Here's how the part is built. I have some questions about the finished solid (model axes, mm). A direction names the side the tool comes from. Give positions to 0.01 mm unless a question says otherwise; leave off trailing zeros. Loops run counter-clockwise (first coordinate to the right, second up) from the corner with the lowest first, then second, coordinate; pieces in that order, holes last. Notation, with made-up numbers: M -12,18 L 33,18 A21 ccw 33,30 Z; hole C -10,-20.5 d7. An arc over 180 degrees is marked long. Write item = value, one per line. Start each with the question number.
Autodesk Inventor part; units mm, degrees
ref_plane "YZ Plane" through (0, 0, 0) normal (1, 0, 0) x (0, 1, 0)
ref_plane "XZ Plane" through (0, 0, 0) normal (0, 1, 0) x (-1, 0, 0)
ref_plane "XY Plane" through (0, 0, 0) normal (0, 0, 1) x (1, 0, 0)
sketch "Sketch1" plane through (0, 0, 0) normal (0, 0, 1) x (1, 0, 0)
  line L0 (-15.5, -9) -> (15.5, -9)
  line L1 (15.5, -9) -> (15.5, 9)
  line L2 (15.5, 9) -> (-15.5, 9)
  line L3 (-15.5, 9) -> (-15.5, -9)
  line L4 (-15.5, -9) -> (15.5, 9) construction
  line L5 (15.5, -9) -> (-15.5, 9) construction
  point P0 (0, 0)
  dimension "d0" = 31
  dimension "d1" = 18
extrude "Extrusion1" add sketch "Sketch1" along normal blind 12.5
sketch "Sketch8" plane through (-15.5, -9, 0) normal (0, -1, 0) x (1, 0, 0)
  circle A0 centre (15.5, 0) radius 7.5
  dimension "d57" = 15
extrude "Extrusion8" cut sketch "Sketch8" against normal through all
sketch "Sketch9" plane through (0, 0, 12.5) normal (0, 0, 1) x (1, 0, 0)
  line L0 (-15.5, -9) -> (15.5, -9)
  point P0 (0, 0)
  point P1 (-11.5, 0)
  point P2 (11.5, 0)
  dimension "d68" = 11.5
  dimension "d69" = 11.5
  dimension "d70" = 9
  dimension "d71" = 9
hole "Hole1" at (-11.5, 0, 12.5) at (11.5, 0, 12.5) direction (0, 0, -1) diameter 4.3 end through all
sketch "Sketch10" plane through (-15.5, -9, 12.5) normal (0, -1, 0) x (1, 0, 0)
  arc A0 (23, -12.5) -> (8, -12.5) centre (15.5, -12.5) ccw
  circle A1 centre (15.5, -12.5) radius 8.5
  dimension "d79" = 17
extrude "Extrusion10" cut sketch "Sketch10" against normal blind 9
properties part number "Colimador superior"
Q1. We'd pull the mould along Y, two halves only. Please class faces 1 (the flat face through (0, -9, 9)), 2 (the flat face through (0, 0, 12.5)), 3 (the cylindrical face through (11.41, 2.15, 6.16)): pulls with the +Y half, pulls with the -Y half, needs draft (parallel to the pull), parting line crosses it, or undercut.
Q2. If I drill on line 1 along X through (y, z) = (-0.75, 3.5); line 2 along X through (y, z) = (0.75, 0.75); line 3 along Y through (x, z) = (11.5, 4.5), over which ranges is the centre line in solid material (lowest first)?
Q3. If we section it at A-A, the plane z = 5.25: List the corners of the cut face in (x, y) for me.
Q4. If we section it at C-C, the plane z = 10.5: List the corners of the cut face in (x, y) for me.
Q5. On a 3-axis mill with a long thin cutter (end or side, diameter ignored), from which of +Z, -Z, +X, -X, +Y, -Y can I reach the whole of each face in a straight line? I mean faces 4 (the flat face through (0, 9, 8)), 5 (the cylindrical face through (0.187, -4.563, 8.498)). Say none if no direction works.
Q6. Will these pins go through, and if not, where does the flat tip stop? pin 1 (4 mm diameter, centred on x = 0, z = 6, fed in from -Y); pin 2 (6 mm diameter, centred on x = 3, y = -0.5, fed in from -Z); pin 3 (2.5 mm diameter, centred on x = 11.5, y = 0, fed in from -Z).
Q7. If we section it at B-B, the plane x = -11.5: List the corners of the cut face in (y, z) for me.
Q8. If we section it at D-D, the plane y = -7: List the corners of the cut face in (x, z) for me, then the cut area to 3 significant figures.
Resolved:
q1.face_1 = pulls with the -Y half
q1.face_2 = needs draft
q1.face_3 = undercut
q2.line_1 = -15.5 to -13.51, -9.49 to -7.75, 7.75 to 9.49, 13.51 to 15.5
q2.line_2 = -15.5 to -13.51, -9.49 to -7.46, 7.46 to 9.49, 13.51 to 15.5
q2.line_3 = -9 to -2.15, 2.15 to 9
q3.outline = M -15.5,-9 L -6.68,-9 L -6.68,0 L -5.36,0 L -5.36,9 L -15.5,9 Z; M 5.36,0 L 6.68,0 L 6.68,-9 L 15.5,-9 L 15.5,9 L 5.36,9 Z; hole C -11.5,0 d4.3; hole C 11.5,0 d4.3
q4.outline = M -15.5,-9 L 15.5,-9 L 15.5,9 L -15.5,9 Z; hole C -11.5,0 d4.3; hole C 11.5,0 d4.3
q5.face_4 = +Z, -Z, +X, -X, +Y
q5.face_5 = -Z, -Y
q6.pin_1 = 0
q6.pin_2 = 4.56
q6.pin_3 = through
q7.outline = M -9,0 L -2.15,0 L -2.15,12.5 L -9,12.5 Z; M 2.15,0 L 9,0 L 9,12.5 L 2.15,12.5 Z
q8.outline = M -15.5,0 L -8.5,0 A8.5 cw 8.5,0 L 15.5,0 L 15.5,12.5 L -15.5,12.5 Z
q8.area = 274 mm²
